Build history of the part. All positions in model axes, mm. A direction names the side the tool comes from. Give positions to 0.01 mm unless a question says otherwise; leave off trailing zeros. Order: outer loops, then holes, each group sorted by start corner. A loop starts at its lowest first (then second) coordinate and runs counter-clockwise, first axis right, second up. Notation, with made-up numbers: M 50.25,-13.5 L 92.25,-13.5 A21 cw 92.25,13.5 Z; hole C 42,37 d11. An arc over 180 degrees is marked long. One line per item, written item: value.
from build123d import *

# Parameters (mm, degrees)
F0_W     = 13.8
F0_H     = 13.8
F1_DEPTH = 9
F2_W     = 5.4
F2_H     = 5.4
F3_DEPTH = 9.001
F4_W     = 11.4
F4_H     = 11.4
F5_DEPTH = 6
F6_R     = 2
F7_R     = 1.5


with BuildPart() as f1:
    # F0 (on Front) → F1 (new body)
    with BuildSketch(Plane.XZ):
        Rectangle(F0_W, F0_H)
    extrude(amount=F1_DEPTH)

    # F2 (on Front) → F3 (cut, through all)
    with BuildSketch(Plane.XZ):
        Rectangle(F2_W, F2_H)
    extrude(amount=F3_DEPTH, mode=Mode.SUBTRACT)

    # F4 (on face) → F5 (cut)
    with BuildSketch(Plane.XZ.offset(9)):
        Rectangle(F4_W, F4_H)
    extrude(amount=-F5_DEPTH, mode=Mode.SUBTRACT)

    # F6
    f6_edges = [f1.edges().sort_by_distance(p)[0] for p in [
        (-6.9, -4.5, 6.9),
        (-6.9, -4.5, -6.9),
        (6.9, -4.5, 6.9),
        (6.9, -4.5, -6.9),
    ]]
    fillet(f6_edges, radius=F6_R)

    # F7
    f7_edges = [f1.edges().sort_by_distance(p)[0] for p in [
        (-5.7, -6, 5.7),
        (5.7, -6, 5.7),
        (-5.7, -6, -5.7),
        (5.7, -6, -5.7),
    ]]
    fillet(f7_edges, radius=F7_R)


solid = f1.part
1) Saw through at D-D, the plane z = -3. Write the cut outline in (x, y).
Check values:
outline: M -6.9,-9 L -5.7,-9 L -5.7,-3 L 5.7,-3 L 5.7,-9 L 6.9,-9 L 6.9,0 L -6.9,0 Z
2) Tool access for faces 1 (the face through (0, -4, 6.9)), 2 (the face through (0, -1, -2.7)), 3 (the face through (5.7, -6, 0)): list every direction of +Z, -Z, +X, -X, +Y, -Y with a clear straight run to the whole face (end or side of a thin tool).
Check values:
face 1: +Z, +X, -X, +Y, -Y
face 2: +Y, -Y
face 3: -Y
3) Drill centre lines: probe 1 along Z at (x, y) = (0.75, -2.5); probe 2 along Z at (x, y) = (-3, -7). Where is each one in solid material? Low to high. Write a range as from..to.
Check values:
probe 1: -6.9..-2.7, 2.7..6.9
probe 2: -6.9..-5.7, 5.7..6.9
4) Saw through at A-A, the plane x = 0.5. Write the cut outline in (y, z), then the cut area to 3 significant figures.
Check values:
outline: M -9,-6.9 L 0,-6.9 L 0,-2.7 L -3,-2.7 L -3,-5.7 L -9,-5.7 Z; M -9,5.7 L -3,5.7 L -3,2.7 L 0,2.7 L 0,6.9 L -9,6.9 Z
area: 39.6 mm^2
5) Mould opens along X. For faces 4 (the face through (-2.7, -1, 0)), 5 (the face through (-6.33, -4.56, 6.3)), 6 (the face through (0, -4, -6.9)) say: released by +X, released by -X, zero draft, split by the parting line, or undercut.
Check values:
face 4: undercut
face 5: released by -X
face 6: zero draft
6) Saw through at C-C, the plane z = -1.5. Write the cut outline in (x, y).
Check values:
outline: M -6.9,-9 L -5.7,-9 L -5.7,-3 L -2.7,-3 L -2.7,0 L -6.9,0 Z; M 2.7,-3 L 5.7,-3 L 5.7,-9 L 6.9,-9 L 6.9,0 L 2.7,0 Z
7) Saw through at B-B, the plane y = -8.25. Write the cut outline in (x, z).
Check values:
outline: M -6.9,-4.9 A2 ccw -4.9,-6.9 L 4.9,-6.9 A2 ccw 6.9,-4.9 L 6.9,4.9 A2 ccw 4.9,6.9 L -4.9,6.9 A2 ccw -6.9,4.9 Z; hole M -5.7,-4.2 A1.5 ccw -4.2,-5.7 L 4.2,-5.7 A1.5 ccw 5.7,-4.2 L 5.7,4.2 A1.5 ccw 4.2,5.7 L -4.2,5.7 A1.5 ccw -5.7,4.2 Z
